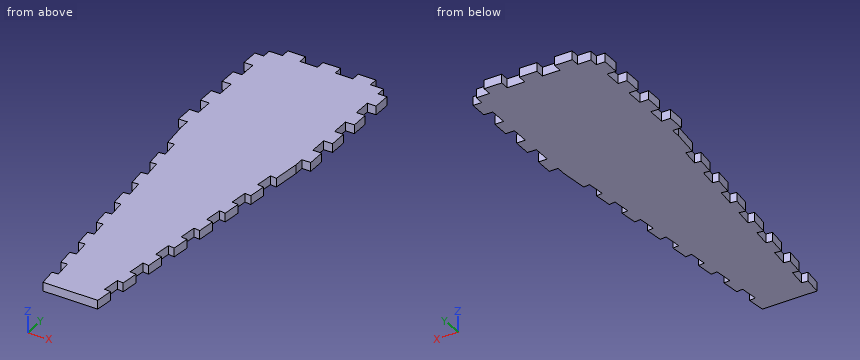
```python
from build123d import *

# Parameters (mm, degrees)
SKETCH1_W           = 95.25
SKETCH1_H           = 304.8
BOSS_EXTRUDE1_DEPTH = 6.35
CUT_EXTRUDE1_DEPTH  = 7.35
SKETCH3_W           = 6.35
SKETCH3_H           = 12.7
CUT_EXTRUDE2_DEPTH  = 7.35
SKETCH4_W           = 9.525
SKETCH4_H           = 6.35
SKETCH4_W_2         = 12.7
CUT_EXTRUDE3_DEPTH  = 7.35
CUT_EXTRUDE4_DEPTH  = 7.35
LPATTERN2_COUNT     = 7
LPATTERN2_PITCH     = 25.4
CUT_EXTRUDE5_DEPTH  = 7.35
LPATTERN3_COUNT     = 7
LPATTERN3_PITCH     = 25.4
SKETCH9_W           = 6.35
SKETCH9_H           = 57.814016323
BOSS_EXTRUDE2_DEPTH = 6.35
LPATTERN4_COUNT     = 5
LPATTERN4_PITCH     = 25.4


with BuildPart() as part:
    # Sketch1 → Boss-Extrude1 (new body)
    with BuildSketch(Plane.XY):
        with Locations((47.625, 152.4)):
            Rectangle(SKETCH1_W, SKETCH1_H)
    extrude(amount=BOSS_EXTRUDE1_DEPTH)

    # Sketch2 → Cut-Extrude1 (cut, through all)
    with BuildSketch(Plane.XY.offset(6.35)):
        Polygon((0, 254), (27.898079092, 0), (0, 0), align=None)
        Polygon((67.351920908, 0), (95.25, 0), (95.25, 254), align=None)
    extrude(amount=-CUT_EXTRUDE1_DEPTH, mode=Mode.SUBTRACT)

    # Sketch3 → Cut-Extrude2 (cut, through all)
    with BuildSketch(Plane.XY.offset(6.35)):
        with Locations((3.175, 298.45)):
            Rectangle(SKETCH3_W, SKETCH3_H)
        with Locations((92.075, 298.45)):
            Rectangle(SKETCH3_W, SKETCH3_H)
    cut_extrude2 = extrude(amount=-CUT_EXTRUDE2_DEPTH, mode=Mode.SUBTRACT)

    # Sketch4 → Cut-Extrude3 (cut, through all)
    with BuildSketch(Plane.XY.offset(6.35)):
        with Locations((11.1125, 301.625)):
            Rectangle(SKETCH4_W, SKETCH4_H)
        with Locations((34.925, 301.625)):
            Rectangle(SKETCH4_W_2, SKETCH4_H)
        with Locations((60.325, 301.625)):
            Rectangle(SKETCH4_W_2, SKETCH4_H)
        with Locations((84.1375, 301.625)):
            Rectangle(SKETCH4_W, SKETCH4_H)
    extrude(amount=-CUT_EXTRUDE3_DEPTH, mode=Mode.SUBTRACT)

    # Sketch5 → Cut-Extrude4 (cut, through all)
    with BuildSketch(Plane.XY.offset(6.35)):
        Polygon((26.511513632, 12.624081599), (25.124948171, 25.248163198), (29.601595278, 25.739855541), (30.988160739, 13.115773942), align=None)
    cut_extrude4 = extrude(amount=-CUT_EXTRUDE4_DEPTH, mode=Mode.SUBTRACT)

    # LPattern2: Cut-Extrude4 ×7
    with Locations(*[Vector(-0.109178383, 0.994022173, 0) * (i * LPATTERN2_PITCH) for i in range(1, LPATTERN2_COUNT)]):
        add(cut_extrude4, mode=Mode.SUBTRACT)

    # Sketch6 → Cut-Extrude5 (cut, through all)
    with BuildSketch(Plane.XY.offset(6.35)):
        Polygon((68.738486368, 12.624081599), (70.125051829, 25.248163198), (65.648404722, 25.739855541), (64.261839261, 13.115773942), align=None)
    cut_extrude5 = extrude(amount=-CUT_EXTRUDE5_DEPTH, mode=Mode.SUBTRACT)

    # LPattern3: Cut-Extrude5 ×7
    with Locations(*[Vector(0.109178383, 0.994022173, 0) * (i * LPATTERN3_PITCH) for i in range(1, LPATTERN3_COUNT)]):
        add(cut_extrude5, mode=Mode.SUBTRACT)

    # Sketch9 → Boss-Extrude2 (add, through all)
    with BuildSketch(Plane.XY.offset(6.35)):
        with Locations((3.175, 225.092991839)):
            Rectangle(SKETCH9_W, SKETCH9_H)
        with Locations((92.075, 225.092991839)):
            Rectangle(SKETCH9_W, SKETCH9_H)
    extrude(amount=-BOSS_EXTRUDE2_DEPTH)

    # LPattern4: Cut-Extrude2 ×5
    with Locations(*[(0, -i * LPATTERN4_PITCH, 0) for i in range(1, LPATTERN4_COUNT)]):
        add(cut_extrude2, mode=Mode.SUBTRACT)


solid = part.part
```
Source: CAD feature listing. Evaluate the final solid. Frame: model axes, mm. Give positions to 0.01 mm unless a question says otherwise; leave off trailing zeros. Order: outer loops, then holes, each group sorted by start corner. A loop starts at its lowest first (then second) coordinate and runs counter-clockwise, first axis right, second up.
(1) Section query A-A (y = 200). Return the cut outline in (x, z), plus the area to 3 significant figures.
(2) Section query B-B (x = 59). Return the cut outline in (y, z), plus the area to 3 significant figures.
(3) Contact query for flat-ended pins moving along their axis: P1, Ø3, axis at y = 223.5, z = 3.5, coming from the -X side; P2, Ø3, axis at y = 36, z = 1, coming from the +X side; P3, Ø1.9, axis at y = 224, z = 4, coming from the +X side; P4, Ø1, axis at x = 69.5, y = 260.5, coming from the -Z side. Output: stop coordinate, or through.
(4) Material intervals for line 1 along Y through (x, z) = (5.5, 3.25); line 2 along Y through (x, z) = (34, 5.75); line 3 along X through (y, z) = (244.5, 2.25), sorted ascending.
Outcome:
1. outline: (6.35, 0) - (88.9, 0) - (88.9, 6.35) - (6.35, 6.35) - close
1. area: 524 mm2
2. outline: (0, 0) - (298.45, 0) - (298.45, 6.35) - (0, 6.35) - close
2. area: 1,900 mm2
3. P1: stops at x = 6.35
3. P2: stops at x = 71.47
3. P3: stops at x = 88.9
3. P4: stops at z = 0
4. line 1: y = 203.2 to 215.9, 228.6 to 241.3, 254 to 266.7, 279.4 to 292.1
4. line 2: y = 0 to 298.45
4. line 3: x = 6.35 to 88.9
